CAD build for the part. Positions are in the model's coordinates, mm. A direction names the side the tool comes from. Give positions to 0.01 mm unless a question says otherwise; leave off trailing zeros. Write each loop counter-clockwise with the first axis right and the second up, starting at its lowest first coordinate (ties: lowest second). Pieces come first, ordered by that corner, then holes. Notation, with made-up numbers: (70, -10) - (109, -10) arc R14 cw to (109, 12) - close; hole circle Ø10 at (76.25, -10.75). An arc over 180 degrees is marked (long way). Put each result on its own line as item: value. Start each with the question number.
1. Tool access for faces 1 (the flat face through (12, 6.629, 8)), 2 (the flat face through (12, -6.629, 8)), 3 (the cylindrical face through (-0.331, -3.006, 2.63)): list every direction of +Z, -Z, +X, -X, +Y, -Y with a clear straight run to the whole face (end or side of a thin tool).
2. Cut at B-B on x = -17. List the corners of the cut face in (y, z), and give its area (3 significant figures).
3. Mould opens along X. For faces 4 (the flat face through (-20.574, 0, -2)), 5 (the flat face through (0, -5, 5.334)), 6 (the flat face through (3.48, 0, 8)) say: +X half, -X half, draft (parallel to the pull), parting line (faces both ways), or undercut.
4. Drop flat-ended pins along their axis: pin 1 (7.5 mm diameter, centred on x = 8.5, z = 9, fed in from -Y); pin 2 (1.4 mm diameter, centred on x = -14, y = 1.5, fed in from +Z); pin 3 (4 mm diameter, centred on x = -0.5, y = -6.5, fed in from +Z). Give the stop position or say it passes through.
5. Cut at A-A on x = 0. List the corners of the cut face in (y, z).
6. Wall check: line 1 (Y direction, x = 10, z = 1.5); line 2 (Z direction, x = -8, y = 3.75); line 3 (Z direction, x = 0, y = -5.75). Give the ranges that are in metal, low to high.
from build123d import *

# Parameters (mm, degrees)
F0_R     = 2.54
F0_R_2   = 1.4097
F0_W     = 17.0942
F0_H     = 13.2588
F1_DEPTH = 4.1275
F2_DEPTH = 15.24
F3_DEPTH = 8.7884
F4_DEPTH = 5.334


with BuildPart() as f1:
    # F0 (on Top) → F1 (new body)
    with BuildSketch(Plane.XY):
        Polygon((20.574, 8.5725), (-20.574, 8.5725), (-20.574, -8.5725), (20.574, -8.5725), (20.574, -6.6294), (3.4798, -6.6294), (3.4798, 6.6294), (20.574, 6.6294), align=None)
        with Locations((0, -5.5245)):
            Circle(F0_R, mode=Mode.SUBTRACT)
        with Locations((-14.097, 2.3495)):
            Circle(F0_R_2, mode=Mode.SUBTRACT)
        with Locations((12.0269, 0)):
            Rectangle(F0_W, F0_H)
        with Locations((0, -5.5245)):
            Circle(F0_R)
        with Locations((-14.097, 2.3495)):
            Circle(F0_R_2)
    extrude(amount=-F1_DEPTH)

    # F0 (on Top) → F2 (join)
    with BuildSketch(Plane.XY):
        with Locations((12.0269, 0)):
            Rectangle(F0_W, F0_H)
    extrude(amount=F2_DEPTH)

    # F0 (on Top) → F3 (join)
    with BuildSketch(Plane.XY):
        with Locations((-14.097, 2.3495)):
            Circle(F0_R_2)
    extrude(amount=F3_DEPTH)

    # F0 (on Top) → F4 (join)
    with BuildSketch(Plane.XY):
        with Locations((0, -5.5245)):
            Circle(F0_R)
    extrude(amount=F4_DEPTH)


solid = f1.part
Report:
1. face 1: +Z, +X, -X, +Y
1. face 2: +Z, +X, -Y
1. face 3: +Z
2. outline: (-8.57, -4.13) - (8.57, -4.13) - (8.57, 0) - (-8.57, 0) - close
2. area: 70.8 mm²
3. face 4: -X half
3. face 5: draft
3. face 6: undercut
4. pin 1: stops at y = -6.63
4. pin 2: stops at z = 8.79
4. pin 3: stops at z = 5.33
5. outline: (-8.57, -4.13) - (8.57, -4.13) - (8.57, 0) - (-2.98, 0) - (-2.98, 5.33) - (-8.06, 5.33) - (-8.06, 0) - (-8.57, 0) - close
6. line 1: y = -6.63 to 6.63
6. line 2: z = -4.13 to 0
6. line 3: z = -4.13 to 5.33
